from build123d import *

# Parameters (mm, degrees)
SKETCH1_R                       = 40.005
EXTRUDE1_DEPTH                  = 18.9992
M5X0_8_TAPPED_HOLE1_D           = 4.2
M5X0_8_TAPPED_HOLE1_DEPTH       = 35.56
M5X0_8_TAPPED_HOLE1_CBORE_D     = 5
M5X0_8_TAPPED_HOLE1_CBORE_DEPTH = 7.62
M5X0_8_TAPPED_HOLE1_TIP         = 1.2618073
HOLE3_D                         = 3.81
HOLE3_DEPTH                     = 6.35
HOLE3_CBORE_D                   = 7.874
HOLE3_CBORE_DEPTH               = 0.254
HOLE3_TIP                       = 1.144639479
CHAMFER1_SIZE                   = 2.54
CIRPATTERN1_COUNT               = 3
SKETCH2_R                       = 38.1
EXTRUDE2_DEPTH                  = 1.00075996


with BuildPart() as part:
    # Sketch1 → Extrude1 (new body)
    with BuildSketch(Plane(origin=(0, 0, 0), x_dir=(1, 0, 0), z_dir=(0, 1, 0))):
        with Locations(Location((0, 0, 0), (0, 0, 270))):  # turned: the seam where the file's is
            Circle(SKETCH1_R)
    extrude(amount=EXTRUDE1_DEPTH)

    # M5x0.8 Tapped Hole1
    with Locations(Plane(origin=(40.005, 6.6802, 0), x_dir=(0, 0, 1), z_dir=(1, 0, 0))):
        with Locations((0, 0)):
            CounterBoreHole(M5X0_8_TAPPED_HOLE1_D / 2, M5X0_8_TAPPED_HOLE1_CBORE_D / 2, M5X0_8_TAPPED_HOLE1_CBORE_DEPTH, depth=M5X0_8_TAPPED_HOLE1_DEPTH)
            with Locations((0, 0, -(M5X0_8_TAPPED_HOLE1_DEPTH + M5X0_8_TAPPED_HOLE1_TIP / 2))):  # 118° drill point
                Cone(0, M5X0_8_TAPPED_HOLE1_D / 2, M5X0_8_TAPPED_HOLE1_TIP, mode=Mode.SUBTRACT)

    # Hole3
    with Locations(Plane(origin=(40.005, 6.6802, 0), x_dir=(0, 0, 1), z_dir=(1, 0, 0))):
        with Locations((0, 0)):
            CounterBoreHole(HOLE3_D / 2, HOLE3_CBORE_D / 2, HOLE3_CBORE_DEPTH, depth=HOLE3_DEPTH)
            with Locations((0, 0, -(HOLE3_DEPTH + HOLE3_TIP / 2))):  # 118° drill point
                Cone(0, HOLE3_D / 2, HOLE3_TIP, mode=Mode.SUBTRACT)

    # Chamfer1
    chamfer1_edges = [part.edges().sort_by_distance(p)[0] for p in [
        (0, 18.9992, -40.005),
    ]]
    chamfer(chamfer1_edges, length=CHAMFER1_SIZE)

    # Sketch9 → M3.5x0.6 Tapped Hole1 (revolve, cut)
    with BuildSketch(Plane(origin=(-10.795, 18.9992, 0), x_dir=(0, 0, 1), z_dir=(1, 0, 0))):
        Polygon((0, 0), (0, 10.523247898), (1.45, 9.652), (1.45, 6.35), (1.75, 6.35), (1.75, 0), align=None)
    m3_5x0_6_tapped_hole1 = revolve(axis=Axis((-10.795, 25.3492, 0), (0, -1, 0)), mode=Mode.SUBTRACT)

    # CirPattern1: M3.5x0.6 Tapped Hole1 ×3 about axis
    cirpattern1_axis = Axis((0, 0, 0), (0, 1, 0))
    for i in range(1, CIRPATTERN1_COUNT):
        add(m3_5x0_6_tapped_hole1.rotate(cirpattern1_axis, i * 360 / CIRPATTERN1_COUNT), mode=Mode.SUBTRACT)

    # Sketch2 → Extrude2 (add)
    with BuildSketch(Plane.XZ):
        with Locations(Location((0, 0, 0), (0, 0, 90))):  # turned: the seam where the file's is
            Circle(SKETCH2_R)
    extrude(amount=EXTRUDE2_DEPTH)

    # Sketch11 → Cut-Revolve1 (revolve, cut)
    with BuildSketch(Plane.XY, mode=Mode.PRIVATE) as cut_revolve1_sk:
        with BuildLine():
            Line((0, 18.9992), (0, 12.7508))
            Line((0, 12.7508), (2.3876, 12.7508))
            Line((2.3876, 12.7508), (2.3876, 13.461592815))
            ThreePointArc((2.3876, 13.461592815), (5.227368483, 15.64396059), (6.480118517, 18.9992))
            Line((6.480118517, 18.9992), (0, 18.9992))
        make_face()
    revolve(cut_revolve1_sk.sketch.rotate(Axis((0, 20.578481537, 0), (0, -1, 0)), 90), axis=Axis((0, 20.578481537, 0), (0, -1, 0)), mode=Mode.SUBTRACT)  # turned: the seam where the file's is


solid = part.part
Could you check a few things on this model? Use its own coordinates, in mm. A direction names the side the tool comes from. Give positions to 0.01 mm unless a question says otherwise; leave off trailing zeros. Order: outer loops, then holes, each group sorted by start corner. A loop starts at its lowest first (then second) coordinate and runs counter-clockwise, first axis right, second up.
Item 1: For faces 4 (the face through (36.12, 9.12, -0.54)), 5 (the face through (23.183, -0.493, -30.235)), 6 (the face through (-12.53, 15.87, -0.23)), which set-ups out of +Z, -Z, +X, -X, +Y, -Y let a thin tool reach every point of the face, with its end or its side?
Item 2: If we section it at B-B, the plane y = 1.75: Write out the boundary of the cut face in (x, z) (3 decimals), plus the area to 3 significant figures.
Item 3: I need wall thicknesses on line 1 (X direction, y = 12.95, z = 0) (3 decimals); line 2 (X direction, y = 11.9, z = 0) (3 decimals); line 3 (X direction, y = 5, z = -24.5). Which ranges of each line are inside material? Lowest first, please.
Item 4: If we mould it in two halves opening along Y, with no side actions, what happens to faces 1 (the face through (-8, 18.999, -1)), 2 (the face through (39.751, 7, 3)), 3 (the face through (-9.38, 11.02, -0.31))? For each: pulls with the +Y half, pulls with the -Y half, needs draft (parallel to the pull), parting line crosses it, or undercut.
Item 5: I'm going to push flat-ended pins straight in: pin 1 (3 mm diameter, centred on y = 16.5, z = 26.5, fed in from -X); pin 2 (4 mm diameter, centred on x = 0.5, z = -1, fed in from +Y); pin 3 (3 mm diameter, centred on x = 10.5, y = 8, fed in from +Z). Where does each tip first touch, or does it pass through?
Item 6: If we section it at A-A, the plane x = 0: Write out the boundary of the cut face in (y, z) (3 decimals), plus the area to 3 significant figures.
Values:
1. face 4: +X
1. face 5: -Y
1. face 6: +Y
2. outline: circle Ø80.01 at (0, 0)
2. area: 5,030 mm2
3. line 1: x = -40.005 to -12.545, -9.045 to -2.388, 2.388 to 40.005
3. line 2: x = -40.005 to -12.245, -9.345 to 40.005
3. line 3: x = -31.63 to 31.63
4. face 1: pulls with the +Y half
4. face 2: undercut
4. face 3: needs draft
5. pin 1: stops at x = -31.23
5. pin 2: stops at y = 13.8
5. pin 3: stops at z = 38.98
6. outline: (-1.001, -38.1) - (0, -38.1) - (0, -40.005) - (16.459, -40.005) - (18.999, -37.465) - (18.999, -6.48) arc R6.5 cw to (13.462, -2.388) - (12.751, -2.388) - (12.751, 2.388) - (13.462, 2.388) arc R6.5 cw to (18.999, 6.48) - (18.999, 37.465) - (16.459, 40.005) - (0, 40.005) - (0, 38.1) - (-1.001, 38.1) - close
6. area: 1,530 mm2
